Read the model definition and answer for the solid it produces. Units are mm, in the model's axes. Round coordinates to 2 decimals unless told otherwise and drop trailing zeros. Write each loop counter-clockwise with the first axis right and the second up, starting at its lowest first coordinate (ties: lowest second). Pieces come first, ordered by that corner, then holes. Notation, with made-up numbers: M 37,33.5 L 82,33.5 A22 ccw 82,68.5 Z; hole C 38,82.25 d2. An arc over 180 degrees is marked long. Use one line per item in the form item = value. Start each with the question number.
Autodesk Inventor part; units mm, degrees
ref_plane "YZ Plane" through (0, 0, 0) normal (1, 0, 0) x (0, 1, 0)
ref_plane "XZ Plane" through (0, 0, 0) normal (0, 1, 0) x (-1, 0, 0)
ref_plane "XY Plane" through (0, 0, 0) normal (0, 0, 1) x (1, 0, 0)
sketch "Sketch1" plane through (0, 0, 0) normal (0, 0, 1) x (1, 0, 0)
  circle A0 centre (0, 0) radius 60
  dimension "d0" = 120
extrude "Extrusion1" add sketch "Sketch1" along normal blind 3
chamfer "Chamfer2" distance 0.5 angle 45 2 edges at (-60, 0, 3) (-60, 0, 0)
sketch "Sketch5" plane through (0, 0, 3) normal (0, 0, 1) x (1, 0, 0)
  circle A0 centre (0, 0) radius 21.05
  dimension "d36" = 42.1
extrude "Extrusion5" cut sketch "Sketch5" against normal through all
chamfer "Chamfer3" distance 3 angle 45 1 edges at (-21.05, 0, 0)
properties part number "spool_side"
Q1. For a pull along Y with two mould halves and no side action, classify faces 1 (the face through (26, 1, 3)), 2 (the face through (11.42, -17.91, 2.81)), 3 (the face through (-59.94, -2.64, 1.49)) as +Y half, -Y half, draft (parallel to the pull), parting line (faces both ways), or undercut.
Q2. Find section C-C on z = 2. Write down the section's boundary in (x, y), and give its area (3 significant figures).
Q3. This flat-tipped pin is pushed along its axis until it touches: pin 1 Ø1 at (y, z) = (19.5, 2.5) entering from +X. Where does it stop, or does it pass through?
Q4. Straight lines are drawn through the part: line 1 (X direction, y = 2, z = 2.45); line 2 (X direction, y = -15, z = 1.3); line 3 (Y direction, x = 12.5, z = 0.1). For each, find the intervals that lie inside material, in ascending order. Write a range as [from, to].
Response:
q1.face_1 = draft
q1.face_2 = undercut
q1.face_3 = parting line
q2.outline = C 0,0 d120; hole C 0,0 d44.1
q2.area = 9,780 mm²
q3.pin_1 = 56.91
q4.line_1 = [-59.97, -21.51], [21.51, 59.97]
q4.line_2 = [-58.09, -17.1], [17.1, 58.09]
q4.line_3 = [-58.27, -20.43], [20.43, 58.27]
